Answer from the drawing. Dimensions are ordinates in mm from the lowest x, y and z of the part. Coordinates: 2 decimals unless noted, no trailing zeros. Loops run counter-clockwise (first coordinate to the right, second up) from the corner with the lowest first, then second, coordinate; pieces in that order, holes last. Notation, with made-up numbers: (0, 55.25) - (22, 55.25) arc R12 ccw to (22, 61.25) - close; hole circle Ø4 at (37.25, 16). An arc over 180 degrees is marked (long way). One line per question, with ' | ' between items. Start each with the question number.
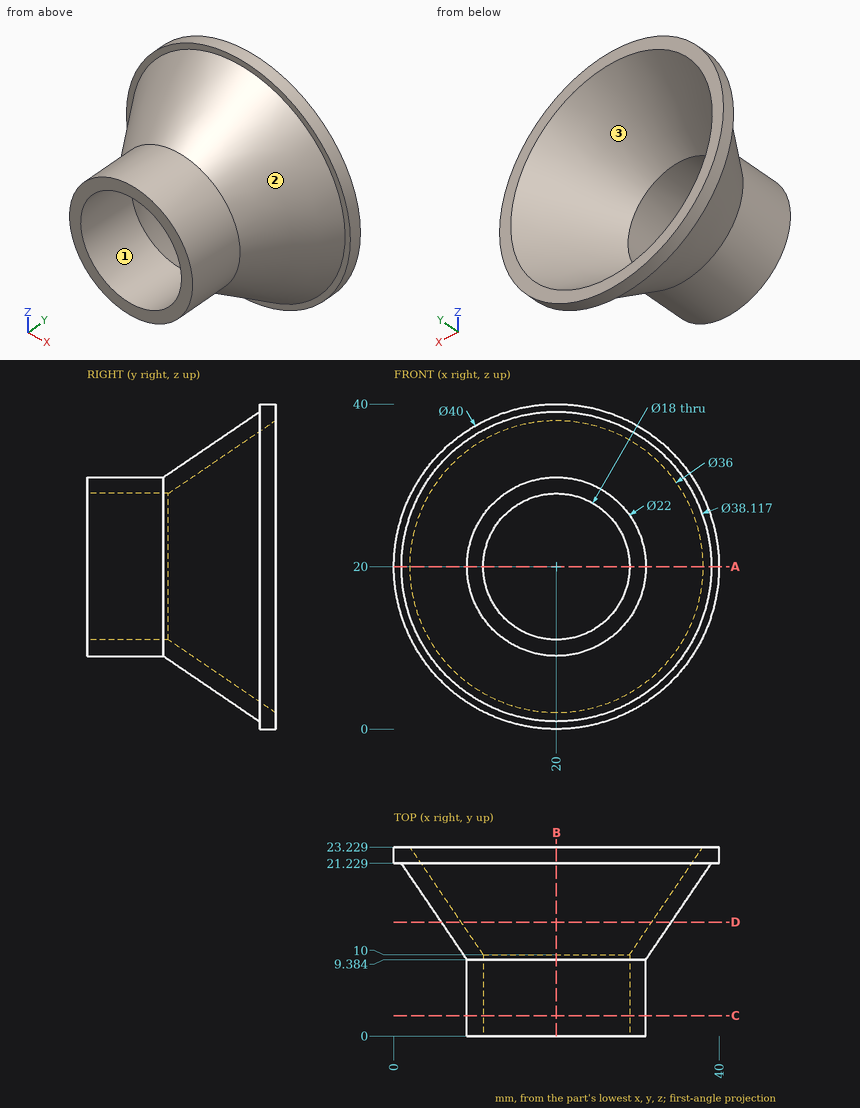
1) The part is cut by section C-C on y = 2.5. Write down the section's boundary in (x, z), and give its area (3 significant figures).
2) The part is cut by section A-A on z = 20. Write down the section's boundary in (x, y).
3) Given pin 1 Ø6 at (y, z) = (8, 14.5) entering from +X; pin 2 Ø1.5 at (y, z) = (2.5, 28.5) entering from +X (1 decimal); pin 3 Ø5 at (y, z) = (4, 21) entering from +X, each flat-ended and moving along its own axis, determine where each tip first touches the part or whether it passes through.
4) The mould has two halves that part along X. Classify the marked faces 1, 2 and 3: released by +X, released by -X, zero draft, split by the parting line, or undercut.
5) Find the intervals of material crossed by line 1 along X through (y, z) = (5.5, 20); line 2 along Y through (x, z) = (11.5, 37.5); line 3 along Z through (x, y) = (5, 21.5) (1 decimal), in increasing order. Write a range as from..to.
6) The part is cut by section B-B on x = 20. Write down the section's boundary in (y, z), and give its area (3 significant figures).
7) The part is cut by section D-D on y = 14. Write down the section's boundary in (x, z).
Answer below:
1) outline: circle Ø22 at (20, 20); hole circle Ø18 at (20, 20) | area: 126 mm2
2) outline: (0, 21.23) - (0.94, 21.23) - (9, 9.38) - (9, 0) - (11, 0) - (11, 10) - (2, 23.23) - (0, 23.23) - close; (29, 0) - (31, 0) - (31, 9.38) - (39.06, 21.23) - (40, 21.23) - (40, 23.23) - (38, 23.23) - (29, 10) - close
3) pin 1: x = 31.13 | pin 2: x = 27.8 | pin 3: x = 31
4) face 1: undercut | face 2: split by the parting line | face 3: undercut
5) line 1: 9..11, 29..31 | line 2: 21.23..23.23 | line 3: 6.8..12.4, 27.6..33.2
6) outline: (0, 9) - (9.38, 9) - (21.23, 0.94) - (21.23, 0) - (23.23, 0) - (23.23, 2) - (10, 11) - (0, 11) - close; (0, 29) - (10, 29) - (23.23, 38) - (23.23, 40) - (21.23, 40) - (21.23, 39.06) - (9.38, 31) - (0, 31) - close | area: 105 mm2
7) outline: circle Ø28.28 at (20, 20); hole circle Ø23.44 at (20, 20)
